Autodesk Inventor part; units mm, degrees
ref_plane "YZ Plane" through (0, 0, 0) normal (1, 0, 0) x (0, 1, 0)
ref_plane "XZ Plane" through (0, 0, 0) normal (0, 1, 0) x (-1, 0, 0)
ref_plane "XY Plane" through (0, 0, 0) normal (0, 0, 1) x (1, 0, 0)
sketch "Sketch1" plane through (0, 0, 0) normal (1, 0, 0) x (0, 1, 0)
  circle A0 centre (0, 0) radius 9.525
  line L0 (0, 9.525) -> (-25.4, 9.525)
  line L1 (-31.75, 9.525) -> (-31.75, 79.375)
  line L2 (-31.75, 79.375) -> (-25.4, 79.375)
  line L3 (-25.4, 79.375) -> (-25.4, 9.525)
  arc A1 (-31.75, 9.525) -> (0.0899, -9.5246) centre (-0.2457, 26.0482) ccw
  dimension "d0" = 19.05
  dimension "d4" = 25.4
  dimension "d5" = 69.85
  dimension "d6" = 6.35
extrude "Extrusion1" add sketch "Sketch1" along normal blind 28.575
fillet "Fillet1" radius 12.7 1 edges at (14.2875, -25.4, 9.525)
sketch "Sketch2" plane through (28.575, 0, 0) normal (1, 0, 0) x (0, 0, -1)
  line L0 (-9.525, 0) -> (-9.525, -12.7)
  arc A0 (-22.225, -25.4) -> (-9.525, -12.7) centre (-22.225, -12.7) ccw
  line L1 (-22.225, -25.4) -> (-79.375, -25.4)
  line L2 (-79.375, -25.4) -> (-79.375, -31.75)
  line L3 (-79.375, -31.75) -> (-9.525, -31.75)
  arc A1 (-9.525, -31.75) -> (9.5246, 0.0899) centre (-26.0482, -0.2457) ccw
  arc A2 (9.5246, 0.0899) -> (-9.525, 0) centre (0, 0) ccw
hole "Hole1" at (28.575, 0, 0) direction (-1, 0, 0) diameter 12.827 depth 25.4 tip angle 118
sketch "Sketch3" plane through (0, -25.4, 79.375) normal (0, 1, 0) x (1, 0, 0)
  line L0 (0, 57.15) -> (28.575, 57.15)
  line L1 (0, 57.15) -> (0, 0)
  line L2 (0, 0) -> (28.575, 0)
  line L3 (28.575, 57.15) -> (28.575, 0)
  line L4 (7.8105, 3.175) -> (20.7645, 3.175)
  line L5 (20.7645, 3.175) -> (20.7645, 8.255)
  line L6 (20.7645, 8.255) -> (7.8105, 8.255)
  line L7 (7.8105, 8.255) -> (7.8105, 3.175)
  line L8 (7.8105, 19.685) -> (20.7645, 19.685)
  line L9 (20.7645, 19.685) -> (20.7645, 14.605)
  line L10 (20.7645, 14.605) -> (7.8105, 14.605)
  line L11 (7.8105, 14.605) -> (7.8105, 19.685)
  point P0 (0, 79.375)
  dimension "d17" = 12.954
  dimension "d18" = 5.08
  dimension "d19" = 7.8105
  dimension "d20" = 28.575
  dimension "d21" = 3.175
  dimension "d22" = 5.08
  dimension "d23" = 6.35
  dimension "d24" = 12.954
extrude "Extrusion2" cut sketch "Sketch3" against normal blind 25.4 contours L7 L6 L5 L4 | L8 L9 L10 L11
equation "\"d19\" = -0.5 * d17 + 0.5 * d20"
properties part number "WheelIntakeBase3.0"
Verification items for the finished model (mm, model axes). A direction names the side the tool comes from. Coordinates: 2 decimals unless noted, no trailing zeros. Loops run counter-clockwise (first coordinate to the right, second up) from the corner with the lowest first, then second, coordinate; pieces in that order, holes last. Notation, with made-up numbers: (-29, -15.75) - (-14, -15.75) arc R9 cw to (-14, -8.75) - close; hole circle Ø2 at (-35.75, -37.5). An arc over 180 degrees is marked (long way). Answer as a JSON object with one key per item and string values.
(1) Mould release check, pull along Y, two halves, no side actions. Record for faces 6 (the conical face through (0.2, -1.43, 0.32)), 7 (the flat face through (14, -31.75, 44)), 8 (the cylindrical face through (14.09, 9.52, 0.25)), 9 (the flat face through (14, -29, 76.2)): pulls with the +Y half, pulls with the -Y half, needs draft (parallel to the pull), parting line crosses it, or undercut.
Response:
{"face 6": "undercut", "face 7": "pulls with the -Y half", "face 8": "pulls with the +Y half", "face 9": "needs draft"}
(2) Access from +Z, -Z, +X, -X, +Y, -Y to the whole of each face (thin tool, end or side, straight path). Record for faces 1 (the flat face through (20.764, -29, 74)), 2 (the flat face through (28.575, -26, 25)), 3 (the flat face through (14, -6, 9.525)), 4 (the cylindrical face through (15.697, -1.926, -6.117)), 5 (the flat face through (14, -29, 79.375)).
Response:
{"face 1": "+Y, -Y", "face 2": "+Z, -Z, +X, +Y, -Y", "face 3": "+Z, +X, -X, +Y", "face 4": "+X", "face 5": "+Z, +X, -X, +Y, -Y"}
(3) Cross-section at D-D, the plane z = 24. Record the boundary of the cut face in (x, y) (3 decimals), then the cut area to 3 significant figures.
Response:
{"outline": "(0, -31.75) - (28.575, -31.75) - (28.575, -25.4) - (0, -25.4) - close", "area": "181 mm²"}
(4) Scan lines: line 1 along Z through (x, y) = (10.25, 0) (1 decimal); line 2 along Y through (x, z) = (21.25, 36); line 3 along Y through (x, z) = (23, 0) (1 decimal). Record each from-to range of solid material in increasing order.
Response:
{"line 1": "z = -9.5 to -6.4, 6.4 to 9.5", "line 2": "y = -31.75 to -25.4", "line 3": "y = -24.5 to -6.4, 6.4 to 9.5"}
(5) Cross-section at A-A, the plane z = 0. Record the boundary of the cut face in (x, y) (1 decimal).
Response:
{"outline": "(0, -24.5) - (28.6, -24.5) - (28.6, -6.4) - (3.2, -6.4) - (0, -1.1) - close; (0, 1.1) - (3.2, 6.4) - (28.6, 6.4) - (28.6, 9.5) - (0, 9.5) - close"}
(6) Cross-section at B-B, the plane x = 10.25. Count the separate pieces of the cut face and the enclosed holes in it, then the cut area to 3 significant figures.
Response:
{"separate pieces": "3", "enclosed holes": "1", "area": "860 mm²"}
(7) Go/stop test with flat-tipped pins: pin 1 Ø1 at (x, y) = (15.5, -21) entering from +Z; pin 2 Ø3 at (x, z) = (18.5, 55.5) entering from +Y; pin 3 Ø14 at (x, y) = (14, -4.5) entering from +Z (3 decimals). Record where each tip stops, or that it passes through.
Response:
{"pin 1": "stops at z = 13.07", "pin 2": "stops at y = -25.4", "pin 3": "stops at z = 9.525"}
